Input: part model. Units: mm. Frame: model coordinates. A direction names the side the tool comes from. Round coordinates to 2 decimals unless told otherwise and drop trailing zeros. Loops run counter-clockwise (first coordinate to the right, second up) from the corner with the lowest first, then second, coordinate; pieces in that order, holes last. Notation, with made-up numbers: M -37.75,8.5 L -24.75,8.5 A30 ccw -24.75,35.5 Z; hole C 14,-3 d1. An arc over 180 degrees is marked long. Return JSON: item names as keys, results as strings. Group by question number.
1) Section C-C (y = -9.5). Output: boundary loops of the cut face in (x, z).
2) Section A-A (y = 7). Output: boundary loops of the cut face in (x, z).
3) Contact query for flat-ended pins moving along their axis: P1, Ø1.5, axis at y = -5.5, z = 2, coming from the +X side; P2, Ø0.9, axis at x = -45.5, z = 1, coming from the -Y side. Output: stop coordinate, or through.
4) Material intervals for line 1 (X direction, y = 3.5, z = 0.45); line 2 (X direction, y = -6.5, z = 0.45); line 3 (Y direction, x = -39, z = 1.5), sorted ascending. Write a range as from..to.
5) Section B-B (z = 2.35). Output: boundary loops of the cut face in (x, y).
6) Mould query, pull axis X, two halves, no side actions, for faces 1 (the face through (57, 9.46, 2)), 2 (the face through (-40, 9.46, 2)), 3 (the face through (7, -3, 3)), 4 (the face through (-46.737, 9, 2)). Classes: +X half, -X half, draft (parallel to the pull), parting line (faces both ways), or undercut.
7) Access query for faces 5 (the face through (55.263, -6, 2)), 6 (the face through (61, 3.46, 2)), 7 (the face through (-44, 3.46, 2)). Directions: +Z, -Z, +X, -X, +Y, -Y. A direction counts if a zero-diameter tool reaches every point of the face in a straight line with its end or side. Return the directions, or none.
from build123d import *

# Parameters (mm, degrees)
EXTRUDE_1_DEPTH     = 3
SKETCH_2_W          = 100
SKETCH_2_H          = 37
EXTRUDE_2_DEPTH     = 3
SKETCH_3_W          = 5
SKETCH_3_H          = 12
EXTRUDE_3_DEPTH     = 3
SKETCH_4_W          = 3
SKETCH_4_H          = 31
CUT_EXTRUDE_1_DEPTH = 3


with BuildPart() as part:
    # 草圖1 → 填料-伸長1 (new body)
    with BuildSketch(Plane.XY):
        Polygon((49.262888429, -21.540240663), (49.262888429, -18.540240663), (39.262888429, -18.540240663), (39.262888429, -21.540240663), (25.262888429, -21.540240663), (25.262888429, -18.540240663), (15.262888429, -18.540240663), (15.262888429, -21.540240663), (1.262888429, -21.540240663), (1.262888429, -18.540240663), (-8.737111571, -18.540240663), (-8.737111571, -21.540240663), (-22.737111571, -21.540240663), (-22.737111571, -18.540240663), (-32.737111571, -18.540240663), (-32.737111571, -21.540240663), (-41.737111571, -21.540240663), (-41.737111571, -8.040240663), (-38.737111571, -8.040240663), (-38.737111571, 1.959759337), (-41.737111571, 1.959759337), (-41.737111571, 15.459759337), (-32.737111571, 15.459759337), (-32.737111571, 12.459759337), (-22.737111571, 12.459759337), (-22.737111571, 15.459759337), (-8.737111571, 15.459759337), (-8.737111571, 12.459759337), (1.262888429, 12.459759337), (1.262888429, 15.459759337), (15.262888429, 15.459759337), (15.262888429, 12.459759337), (25.262888429, 12.459759337), (25.262888429, 15.459759337), (39.262888429, 15.459759337), (39.262888429, 12.459759337), (49.262888429, 12.459759337), (49.262888429, 15.459759337), (58.262888429, 15.459759337), (58.262888429, 1.959759337), (55.262888429, 1.959759337), (55.262888429, -8.040240663), (58.262888429, -8.040240663), (58.262888429, -21.540240663), align=None)
    extrude(amount=EXTRUDE_1_DEPTH)

    # 草圖2 → 填料-伸長2 (add)
    with BuildSketch(Plane.XY.offset(3)):
        with Locations((8.262888429, -3.040240663)):
            Rectangle(SKETCH_2_W, SKETCH_2_H)
    extrude(amount=-EXTRUDE_2_DEPTH)

    # 草圖3 → 填料-伸長3 (add)
    with BuildSketch(Plane.XY.offset(3)):
        with Locations((60.762888429, 9.459759337)):
            Rectangle(SKETCH_3_W, SKETCH_3_H)
        with Locations((-44.237111571, 9.459759337)):
            Rectangle(SKETCH_3_W, SKETCH_3_H)
    extrude(amount=-EXTRUDE_3_DEPTH)

    # 草圖4 → 除料-伸長1 (cut)
    with BuildSketch(Plane.XY.offset(3)):
        with Locations((-40.237111571, -6.040240663)):
            Rectangle(SKETCH_4_W, SKETCH_4_H)
        with Locations((56.762888429, -6.040240663)):
            Rectangle(SKETCH_4_W, SKETCH_4_H)
    extrude(amount=-CUT_EXTRUDE_1_DEPTH, mode=Mode.SUBTRACT)


solid = part.part
Returned:
{
 "1": {"outline": "M -38.74,0 L 55.26,0 L 55.26,3 L -38.74,3 Z"},
 "2": {"outline": "M -46.74,0 L -41.74,0 L -41.74,3 L -46.74,3 Z; M -38.74,0 L 55.26,0 L 55.26,3 L -38.74,3 Z; M 58.26,0 L 63.26,0 L 63.26,3 L 58.26,3 Z"},
 "3": {"P1": "stops at x = 55.26", "P2": "stops at y = 3.46"},
 "4": {"line 1": "x = -46.74..-41.74, -38.74..55.26, 58.26..63.26", "line 2": "x = -38.74..55.26", "line 3": "y = 9.46..15.46"},
 "5": {"outline": "M -46.74,3.46 L -41.74,3.46 L -41.74,9.46 L -38.74,9.46 L -38.74,-21.54 L 55.26,-21.54 L 55.26,9.46 L 58.26,9.46 L 58.26,3.46 L 63.26,3.46 L 63.26,15.46 L -46.74,15.46 Z"},
 "6": {"face 1": "undercut", "face 2": "undercut", "face 3": "draft", "face 4": "-X half"},
 "7": {"face 5": "+Z, -Z, -Y", "face 6": "+Z, -Z, +X, -Y", "face 7": "+Z, -Z, -X, -Y"}
}
